```python
from build123d import *

# Parameters (mm, degrees)
SKICA1_W                 = 2.5
SKICA1_H                 = 4.9
P_IDAT_VYSUNUT_M1_DEPTH  = 2.5
ODEBRAT_VYSUNUT_M1_DEPTH = 2.5
SKICA4_W                 = 0.9
SKICA4_H                 = 0.9
P_IDAT_VYSUNUT_M2_DEPTH  = 5.9
SKICA5_W                 = 0.9
SKICA5_H                 = 0.9
P_IDAT_VYSUNUT_M3_DEPTH  = 2.8


with BuildPart() as part:
    # Skica1 → Přidat vysunutím1 (new body)
    with BuildSketch(Plane.XY):
        with Locations((-1.25, 2.45)):
            Rectangle(SKICA1_W, SKICA1_H)
    extrude(amount=P_IDAT_VYSUNUT_M1_DEPTH)

    # Skica3 → Odebrat vysunutím1 (cut)
    with BuildSketch(Plane(origin=(0, 0, 0), x_dir=(0, 0, -1), z_dir=(1, 0, 0))):
        Polygon((-2.5, 2.95), (-2, 2.45), (-2.5, 1.95), align=None)
        Polygon((0, 2.95), (-0.5, 2.45), (0, 1.95), align=None)
        Polygon((-2, 4.9), (-2.5, 4.4), (-2.5, 4.9), align=None)
        Polygon((-2.5, 0.5), (-2, 0), (-2.5, 0), align=None)
        Polygon((-0.5, 0), (0, 0.5), (0, 0), align=None)
        Polygon((0, 4.9), (0, 4.4), (-0.5, 4.9), align=None)
    extrude(amount=-ODEBRAT_VYSUNUT_M1_DEPTH, mode=Mode.SUBTRACT)

    # Skica4 → Přidat vysunutím2 (add)
    with BuildSketch(Plane(origin=(0, 0, 0), x_dir=(0, 0, -1), z_dir=(1, 0, 0))):
        with Locations((-1.25, 3.675)):
            Rectangle(SKICA4_W, SKICA4_H)
        with Locations((-1.25, 1.225)):
            Rectangle(SKICA4_W, SKICA4_H)
    extrude(amount=P_IDAT_VYSUNUT_M2_DEPTH)

    # Skica5 → Přidat vysunutím3 (add)
    with BuildSketch(Plane.ZY.offset(2.5)):
        with Locations((1.25, 3.675)):
            Rectangle(SKICA5_W, SKICA5_H)
        with Locations((1.25, 1.225)):
            Rectangle(SKICA5_W, SKICA5_H)
    extrude(amount=P_IDAT_VYSUNUT_M3_DEPTH)


solid = part.part
```
Input: part model. Units: mm. Frame: model coordinates. A direction names the side the tool comes from. Coordinates: 2 decimals unless noted, no trailing zeros. Order: outer loops, then holes, each group sorted by start corner. A loop starts at its lowest first (then second) coordinate and runs counter-clockwise, first axis right, second up. Notation, with made-up numbers: (4, -28.75) - (62, -28.75) arc R12 cw to (62, -6.75) - close; hole circle Ø9 at (41.25, -13.5). An arc over 180 degrees is marked (long way). Return JSON: item names as keys, results as strings.
Q1. First-contact query: pin 1 (0.7 mm diameter, centred on x = 4.5, y = 1.5, fed in from +Z); pin 2 (0.7 mm diameter, centred on x = 1.5, z = 1, fed in from -Y) (3 decimals); pin 3 (1 mm diameter, centred on x = -3.5, y = 1.5, fed in from -Z). Flat tips, straight axial feed; report the tip coordinate or a pass-through.
The answers:
{"pin 1": "stops at z = 1.7", "pin 2": "stops at y = 0.775", "pin 3": "stops at z = 0.8"}
Q2. Draft query along Y for faces 1 (the flat face through (3, 1.675, 1)), 2 (the flat face through (-4, 1.675, 1)), 3 (the flat face through (2.9, 3.7, 1.7)), 4 (the flat face through (-1, 4.9, 1)). Return one class per face: +Y half, -Y half, draft (parallel to the pull), parting line (faces both ways), or undercut.
The answers:
{"face 1": "undercut", "face 2": "undercut", "face 3": "draft", "face 4": "+Y half"}
Q3. Access query for faces 5 (the flat face through (3, 0.775, 1)), 6 (the flat face through (3, 4.125, 1)), 7 (the flat face through (-4, 0.775, 1)), 8 (the flat face through (-4, 1, 0.8)), 9 (the flat face through (3, 1, 1.7)). Directions: +Z, -Z, +X, -X, +Y, -Y. A direction counts if a zero-diameter tool reaches every point of the face in a straight line with its end or side. Return the directions, or none.
The answers:
{"face 5": "+Z, -Z, +X, -Y", "face 6": "+Z, -Z, +X, +Y", "face 7": "+Z, -Z, -X, -Y", "face 8": "-Z, -X, +Y, -Y", "face 9": "+Z, +X, +Y, -Y"}
Q4. Cut plane A-A (z = 2.1). Return loops of the section in (x, y), then the cut area to 4 significant figures.
The answers:
{"outline": "(-2.5, 0.1) - (0, 0.1) - (0, 2.35) - (-2.5, 2.35) - close; (-2.5, 2.55) - (0, 2.55) - (0, 4.8) - (-2.5, 4.8) - close", "area": "11.25 mm2"}
Q5. Cut plane C-C (y = 4). Return loops of the section in (x, z).
The answers:
{"outline": "(-5.3, 0.8) - (-2.5, 0.8) - (-2.5, 0) - (0, 0) - (0, 0.8) - (5.9, 0.8) - (5.9, 1.7) - (0, 1.7) - (0, 2.5) - (-2.5, 2.5) - (-2.5, 1.7) - (-5.3, 1.7) - close"}
Q6. Ray query, probe 1 along X at (y, z) = (1.4, 0.3); probe 2 along Z at (x, y) = (-3.25, 1.6); probe 3 along Z at (x, y) = (-1.75, 4.7). Return the intervals inside material, ascending.
The answers:
{"probe 1": "x = -2.5 to 0", "probe 2": "z = 0.8 to 1.7", "probe 3": "z = 0.3 to 2.2"}
Q7. Cut plane B-B (x = 2). Return loops of the section in (y, z) (3 decimals).
The answers:
{"outline": "(0.775, 0.8) - (1.675, 0.8) - (1.675, 1.7) - (0.775, 1.7) - close; (3.225, 0.8) - (4.125, 0.8) - (4.125, 1.7) - (3.225, 1.7) - close"}
Q8. Cut plane D-D (x = -0.5). Return loops of the section in (y, z), then the cut area to 4 significant figures.
The answers:
{"outline": "(0, 0.5) - (0.5, 0) - (1.95, 0) - (2.45, 0.5) - (2.95, 0) - (4.4, 0) - (4.9, 0.5) - (4.9, 2) - (4.4, 2.5) - (2.95, 2.5) - (2.45, 2) - (1.95, 2.5) - (0.5, 2.5) - (0, 2) - close", "area": "11.25 mm2"}
